Could you check a few things on this drawing? It's one solid part, dimensions in mm from its lowest x, y, z. A direction names the side the tool comes from. Round coordinates to 2 decimals unless told otherwise and drop trailing zeros. Write each loop counter-clockwise with the first axis right and the second up, starting at its lowest first coordinate (ties: lowest second). Pieces come first, ordered by that corner, then holes. Notation, with made-up numbers: (3.25, 84) -> (37.25, 84) arc R17 ccw to (37.25, 91) -> close; hole circle Ø3 at (-20.5, 72.5). An arc over 180 degrees is marked (long way). Return JSON: item names as keys, results as strings.
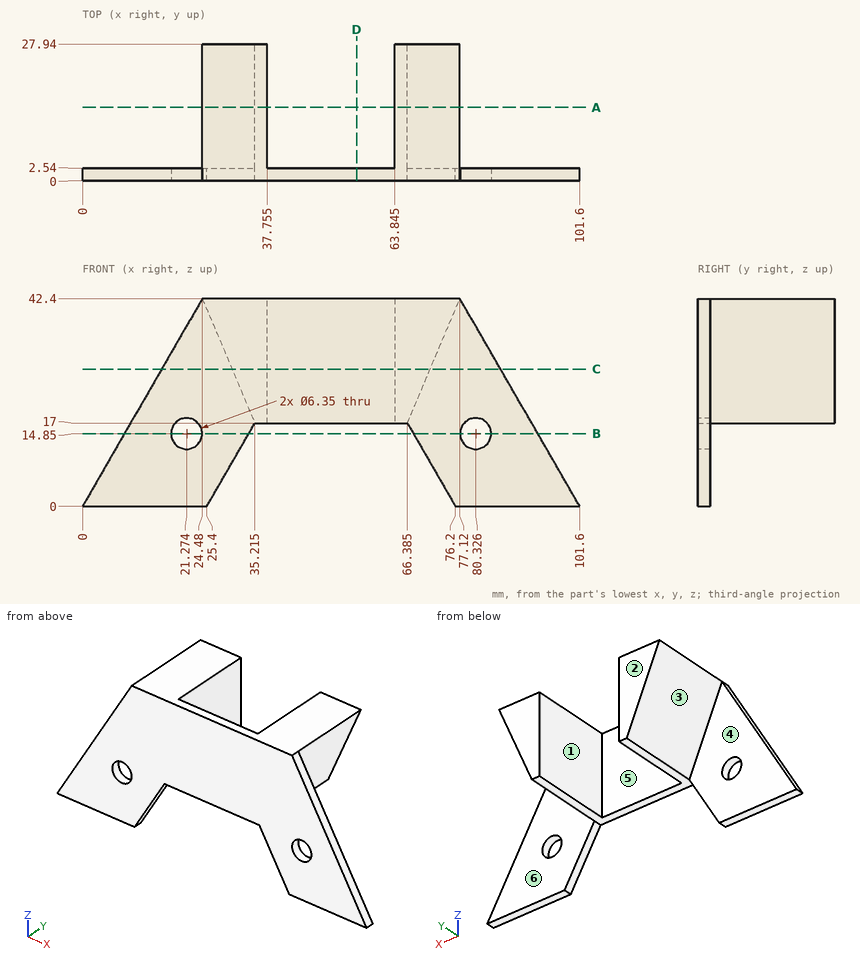
1) I want a section at B-B, the plane z = 14.85. Please give me the cut outline in (x, y).
Return value:
{"outline": "(8.57, 0) -> (18.1, 0) -> (18.1, 2.54) -> (8.57, 2.54) -> close; (24.45, 0) -> (33.97, 0) -> (33.97, 2.54) -> (24.45, 2.54) -> close; (67.63, 0) -> (77.15, 0) -> (77.15, 2.54) -> (67.63, 2.54) -> close; (83.5, 0) -> (93.03, 0) -> (93.03, 2.54) -> (83.5, 2.54) -> close"}
2) If I drill on probe 1 along Y at (x, z) = (22, 19); probe 2 along X at (y, z) = (4.75, 26.5) (1 decimal); probe 3 along Z at (x, y) = (61.5, 1.25), over which ranges is the centre line in solid material (lowest first)? Write a range as [from, to].
Return value:
{"probe 1": "[0, 2.54]", "probe 2": "[31.2, 37.8], [63.8, 70.4]", "probe 3": "[17, 42.4]"}
3) I want a section at A-A, the plane y = 15. Please give me the cut outline in (x, z) (1 decimal), and give its area (3 significant figures).
Return value:
{"outline": "(24.5, 42.4) -> (35.2, 17) -> (37.8, 17) -> (37.8, 42.4) -> close; (63.8, 17) -> (66.4, 17) -> (77.1, 42.4) -> (63.8, 42.4) -> close", "area": "402 mm²"}
4) Will these pins go through, and if not, where does the flat tip stop? pin 1 Ø7.5 at (y, z) = (12, 25.5) entering from +X; pin 2 Ø7.5 at (x, z) = (51, 35) entering from +Y; pin 3 Ø1 at (x, y) = (67, 7.5) entering from -Z.
Return value:
{"pin 1": "x = 71.56", "pin 2": "y = 2.54", "pin 3": "z = 17.27"}
5) I want a section at D-D, the plane x = 56. Please give me the cut outline in (y, z).
Return value:
{"outline": "(0, 17) -> (2.54, 17) -> (2.54, 42.4) -> (0, 42.4) -> close"}
6) Thinking about a two-plate mould opening in X: for the marked faces 1, 2 and 3, which applies, pulls with the +X half, pulls with the -X half, needs draft (parallel to the pull), parting line crosses it, or undercut?
Return value:
{"face 1": "undercut", "face 2": "needs draft", "face 3": "pulls with the -X half"}
7) For the marked faces 4, 5 and 6, which set-ups out of +Z, -Z, +X, -X, +Y, -Y let a thin tool reach every point of the face, with its end or its side?
Return value:
{"face 4": "-Z, -X, +Y", "face 5": "+Z, -Z, +Y", "face 6": "-Z, +X, +Y"}
8) I want a section at C-C, the plane z = 28. Please give me the cut outline in (x, y) (1 decimal), and give its area (3 significant figures).
Return value:
{"outline": "(16.2, 0) -> (85.4, 0) -> (85.4, 2.5) -> (71, 2.5) -> (71, 27.9) -> (63.8, 27.9) -> (63.8, 2.5) -> (37.8, 2.5) -> (37.8, 27.9) -> (30.6, 27.9) -> (30.6, 2.5) -> (16.2, 2.5) -> close", "area": "541 mm²"}
